Part model, mm, in its own coordinate system. Face numbers are marked on the shaded views. A direction names the side the tool comes from. Coordinates: 2 decimals unless noted, no trailing zeros. Loops run counter-clockwise (first coordinate to the right, second up) from the corner with the lowest first, then second, coordinate; pieces in that order, holes last. Notation, with made-up numbers: (17.5, 65) -> (67.5, 65) arc R29 cw to (67.5, 101) -> close; hole circle Ø1 at (-33, -5). An arc over 180 degrees is marked (long way). One line per item, written item: value. Start each with the question number.
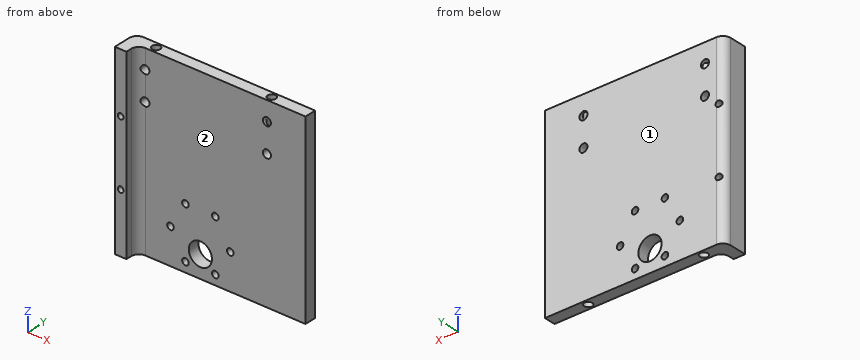
from build123d import *

# Parameters (mm, degrees)
SKETCH1_W           = 93
SKETCH1_H           = 96.2019
SKETCH1_R           = 6
SKETCH1_R_2         = 1.7
SKETCH1_R_3         = 2.1
BOSS_EXTRUDE1_DEPTH = 6
SKETCH2_W           = 6
SKETCH2_H           = 96.2019
SKETCH2_R           = 1.5
BOSS_EXTRUDE2_DEPTH = 7
SKETCH2_3_R         = 1.5
CUT_EXTRUDE2_DEPTH  = 134.988079931
FILLET1_R           = 4
SKETCH3_R           = 2.1
CUT_EXTRUDE3_DEPTH  = 18
CUT_EXTRUDE4_START  = -78.2019
SKETCH3_2_R         = 2.1
CUT_EXTRUDE4_DEPTH  = 18


with BuildPart() as part:
    # Sketch1 → Boss-Extrude1 (new body)
    with BuildSketch(Plane(origin=(0, 0, 0), x_dir=(-1, 0, 0), z_dir=(0, 1, 0))):
        with Locations((46.5, 48.10095)):
            Rectangle(SKETCH1_W, SKETCH1_H)
        with Locations(Location((54.5, 11.5, 0), (0, 0, 90))):
            Circle(SKETCH1_R, mode=Mode.SUBTRACT)
        with Locations(Location((39, 18.5, 0), (0, 0, 90))):
            Circle(SKETCH1_R_2, mode=Mode.SUBTRACT)
        with Locations(Location((46.75, 31.923393759, 0), (0, 0, 90))):
            Circle(SKETCH1_R_2, mode=Mode.SUBTRACT)
        with Locations(Location((62.25, 31.923393759, 0), (0, 0, 90))):
            Circle(SKETCH1_R_2, mode=Mode.SUBTRACT)
        with Locations(Location((70, 18.5, 0), (0, 0, 90))):
            Circle(SKETCH1_R_2, mode=Mode.SUBTRACT)
        with Locations(Location((62.25, 5.076606241, 0), (0, 0, 90))):
            Circle(SKETCH1_R_2, mode=Mode.SUBTRACT)
        with Locations(Location((46.75, 5.076606241, 0), (0, 0, 90))):
            Circle(SKETCH1_R_2, mode=Mode.SUBTRACT)
        with Locations(Location((20, 86.2019, 0), (0, 0, 90))):
            Circle(SKETCH1_R_3, mode=Mode.SUBTRACT)
        with Locations(Location((83, 86.2019, 0), (0, 0, 90))):
            Circle(SKETCH1_R_3, mode=Mode.SUBTRACT)
        with Locations(Location((83, 71.2019, 0), (0, 0, 90))):
            Circle(SKETCH1_R_3, mode=Mode.SUBTRACT)
        with Locations(Location((20, 71.2019, 0), (0, 0, 90))):
            Circle(SKETCH1_R_3, mode=Mode.SUBTRACT)
    extrude(amount=BOSS_EXTRUDE1_DEPTH)

    # Sketch2 → Boss-Extrude2 (add)
    with BuildSketch(Plane(origin=(0, 0, 0), x_dir=(-1, 0, 0), z_dir=(0, -1, 0))):
        with Locations((90, -48.10095)):
            Rectangle(SKETCH2_W, SKETCH2_H)
        with Locations(Location((90, -65.10095, 0), (0, 0, 90))):
            Circle(SKETCH2_R, mode=Mode.SUBTRACT)
        with Locations(Location((90, -31.10095, 0), (0, 0, 90))):
            Circle(SKETCH2_R, mode=Mode.SUBTRACT)
    extrude(amount=BOSS_EXTRUDE2_DEPTH)

    # Sketch2<3> → Cut-Extrude2 (cut, through all)
    with BuildSketch(Plane(origin=(0, 0, 0), x_dir=(-1, 0, 0), z_dir=(0, -1, 0))):
        with Locations(Location((90, -31.10095, 0), (0, 0, 90))):
            Circle(SKETCH2_3_R)
        with Locations(Location((90, -65.10095, 0), (0, 0, 90))):
            Circle(SKETCH2_3_R)
    extrude(amount=-CUT_EXTRUDE2_DEPTH, mode=Mode.SUBTRACT)

    # Fillet1
    # the kernel refuses this fillet: 4 mm, written as the material it adds along each edge
    with BuildSketch(Plane(origin=(-87, 0, 96.2019), x_dir=(0, -1, 0), z_dir=(0, 0, -1))) as fillet1_piece_1_section:
        with BuildLine():
            CenterArc((FILLET1_R, -FILLET1_R), FILLET1_R, 90, 90)
            Line((0, -FILLET1_R), (0, 0))
            Line((0, 0), (FILLET1_R, 0))
        make_face()
    fillet1_piece_1 = extrude(amount=96.2019, mode=Mode.PRIVATE)
    fillet1_piece_1 = fillet1_piece_1 - Plane(origin=(-83, -0.912137569, 71.2019), x_dir=(0, 0, 1), z_dir=(0, -1, 0)) * Cylinder(2.1, 209, mode=Mode.PRIVATE)
    fillet1_piece_1 = fillet1_piece_1 - Plane(origin=(-83, -0.912137569, 86.2019), x_dir=(0, 0, 1), z_dir=(0, -1, 0)) * Cylinder(2.1, 209, mode=Mode.PRIVATE)
    add(fillet1_piece_1)
    # the kernel refuses this fillet: 4 mm, written as the material it takes off along each edge
    with BuildSketch(Plane(origin=(-93, 6, -10), x_dir=(1, 0, 0), z_dir=(0, 0, 1))) as fillet1_2_piece_1:
        with BuildLine():
            CenterArc((FILLET1_R, -FILLET1_R), FILLET1_R, 90, 90)
            Line((0, -FILLET1_R), (0, 0))
            Line((0, 0), (FILLET1_R, 0))
        make_face()
    extrude(amount=116.2019, mode=Mode.SUBTRACT)

    # Sketch3 → Cut-Extrude3 (cut)
    with BuildSketch(Plane(origin=(0, 0, 0), x_dir=(1, 0, 0), z_dir=(0, 0, -1))):
        with Locations(Location((-80, -3, 0), (0, 0, 180))):
            Circle(SKETCH3_R)
        with Locations(Location((-20, -3, 0), (0, 0, 180))):
            Circle(SKETCH3_R)
    extrude(amount=-CUT_EXTRUDE3_DEPTH, mode=Mode.SUBTRACT)

    # Sketch3<2> → Cut-Extrude4 (cut)
    with BuildSketch(Plane(origin=(0, 0, 0), x_dir=(1, 0, 0), z_dir=(0, 0, -1)).offset(CUT_EXTRUDE4_START)):
        with Locations(Location((-80, -3, 0), (0, 0, 180))):
            Circle(SKETCH3_2_R)
        with Locations(Location((-20, -3, 0), (0, 0, 180))):
            Circle(SKETCH3_2_R)
    extrude(amount=-CUT_EXTRUDE4_DEPTH, mode=Mode.SUBTRACT)


solid = part.part
1) Slice it at A-A (x = -54.5). Give the cut face in (y, z).
2) Probe line 1 (Z direction, x = -90, y = -2); line 2 (Y direction, x = -80, z = 85); line 3 (Y direction, x = -48, z = 21). List the from-to ranges inside material, lowest first. Write a range as from..to.
3) Pin check, flat tips, straight feed: pin 1 Ø2.5 at (x, z) = (-20, 71.2) entering from -Y; pin 2 Ø5 at (y, z) = (-5.5, 29) entering from +X; pin 3 Ø4.5 at (x, z) = (-39, 18.5) entering from -Y; pin 4 Ø4 at (x, y) = (-20, 3) entering from -Z. Stop position of each tip, or through.
4) Tool access for the marked faces 1 and 2: list every direction of +Z, -Z, +X, -X, +Y, -Y with a clear straight run to the whole face (end or side of a thin tool).
5) Slice it at D-D (z = 23). Give the cut face in (x, y), then the cut area to 3 significant figures.
6) Slice it at C-C (x = -20). Give the cut face in (y, z).
7) Slice it at B-B (z = 11.5). Give the cut face in (x, y).
Check sheet entries:
1. outline: (0, 0) -> (6, 0) -> (6, 5.5) -> (0, 5.5) -> close; (0, 17.5) -> (6, 17.5) -> (6, 96.2) -> (0, 96.2) -> close
2. line 1: z = 0..29.6, 32.6..63.6, 66.6..96.2
2. line 2: y = 0..0.9, 5.1..6
2. line 3: y = 0..6
3. pin 1: passes through
3. pin 2: stops at x = -86.87
3. pin 3: stops at y = 0
3. pin 4: stops at z = 18
4. face 1: +Z, -Z, +X, -X, +Y
4. face 2: +Z, -Z, +X, -Y
5. outline: (-93, -7) -> (-87, -7) -> (-87, -4) arc R4 cw to (-83, 0) -> (0, 0) -> (0, 6) -> (-89, 6) arc R4 ccw to (-93, 2) -> close
5. area: 600 mm^2
6. outline: (0, 0) -> (0.9, 0) -> (0.9, 18) -> (5.1, 18) -> (5.1, 0) -> (6, 0) -> (6, 69.1) -> (0, 69.1) -> close; (0, 73.3) -> (6, 73.3) -> (6, 84.1) -> (5.1, 84.1) -> (5.1, 78.2) -> (0.9, 78.2) -> (0.9, 84.1) -> (0, 84.1) -> close; (0, 88.3) -> (0.9, 88.3) -> (0.9, 96.2) -> (0, 96.2) -> close; (5.1, 88.3) -> (6, 88.3) -> (6, 96.2) -> (5.1, 96.2) -> close
7. outline: (-93, -7) -> (-87, -7) -> (-87, -4) arc R4 cw to (-83, 0) -> (-60.5, 0) -> (-60.5, 6) -> (-89, 6) arc R4 ccw to (-93, 2) -> close; (-48.5, 0) -> (0, 0) -> (0, 6) -> (-48.5, 6) -> close; hole circle Ø4.2 at (-80, 3); hole circle Ø4.2 at (-20, 3)
